from build123d import *

# Parameters (mm, degrees)
SKETCH_1_W          = 30
SKETCH_1_H          = 30
SKETCH_1_R          = 1.55
EXTRUDE_1_DEPTH     = 10
SKETCH_2_R          = 3.5
CUT_EXTRUDE_1_DEPTH = 3
SKETCH_3_W          = 6
SKETCH_3_H          = 15
EXTRUDE_3_DEPTH     = 3
SKETCH_5_W          = 1.5
SKETCH_5_H          = 0.7
CUT_EXTRUDE_3_DEPTH = 36
SKETCH_6_R          = 3
EXTRUDE_4_DEPTH     = 6


with BuildPart() as part:
    # 草图1 → 凸台-拉伸1 (new body)
    with BuildSketch(Plane(origin=(0, 0, 0), x_dir=(1, 0, 0), z_dir=(0, 1, 0))):
        Rectangle(SKETCH_1_W, SKETCH_1_H)
        with Locations(Location((-5, 5, 0), (0, 0, 270))):
            Circle(SKETCH_1_R, mode=Mode.SUBTRACT)
        with Locations(Location((5, 5, 0), (0, 0, 270))):
            Circle(SKETCH_1_R, mode=Mode.SUBTRACT)
        with Locations(Location((5, -5, 0), (0, 0, 270))):
            Circle(SKETCH_1_R, mode=Mode.SUBTRACT)
        with Locations(Location((-5, -5, 0), (0, 0, 270))):
            Circle(SKETCH_1_R, mode=Mode.SUBTRACT)
    extrude(amount=EXTRUDE_1_DEPTH)

    # 草图2 → 切除-拉伸1 (cut)
    with BuildSketch(Plane.XZ):
        with Locations(Location((-5, 5, 0), (0, 0, 270))):
            Circle(SKETCH_2_R)
        with Locations(Location((5, 5, 0), (0, 0, 270))):
            Circle(SKETCH_2_R)
        with Locations(Location((5, -5, 0), (0, 0, 270))):
            Circle(SKETCH_2_R)
        with Locations(Location((-5, -5, 0), (0, 0, 270))):
            Circle(SKETCH_2_R)
    extrude(amount=-CUT_EXTRUDE_1_DEPTH, mode=Mode.SUBTRACT)

    # 草图3 → 凸台-拉伸3 (add)
    with BuildSketch(Plane.XZ):
        with Locations((-12, 0)):
            Rectangle(SKETCH_3_W, SKETCH_3_H)
        with Locations((12, 0)):
            Rectangle(SKETCH_3_W, SKETCH_3_H)
    extrude(amount=EXTRUDE_3_DEPTH)

    # 草图5 → 切除-拉伸3 (cut, through all)
    with BuildSketch(Plane.ZY.offset(15)):
        with Locations((-6.75, -0.35)):
            Rectangle(SKETCH_5_W, SKETCH_5_H)
        with Locations((6.75, -0.35)):
            Rectangle(SKETCH_5_W, SKETCH_5_H)
    extrude(amount=-CUT_EXTRUDE_3_DEPTH, mode=Mode.SUBTRACT)

    # 草图6 → 凸台-拉伸4 (add)
    with BuildSketch(Plane.XZ):
        with Locations(Location((0, 0, 0), (0, 0, 270))):
            Circle(SKETCH_6_R)
    extrude(amount=EXTRUDE_4_DEPTH)


solid = part.part
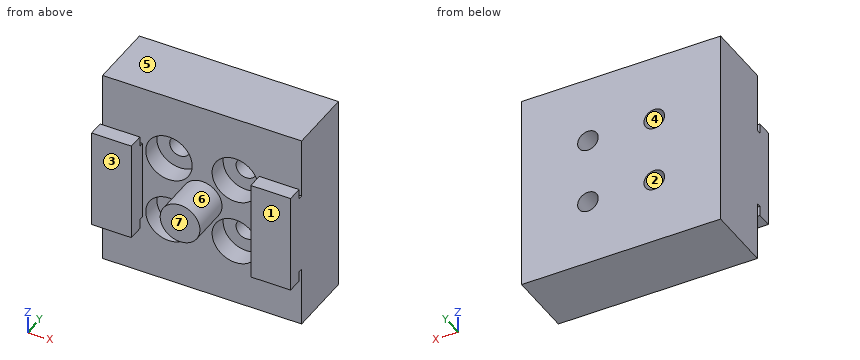
Design review of the part built by this model. Coordinates are the model's own, in mm. Face numbers are marked on the shaded views. A direction names the side the tool comes from. Round coordinates to 2 decimals unless told otherwise and drop trailing zeros. Write each loop counter-clockwise with the first axis right and the second up, starting at its lowest first coordinate (ties: lowest second). Pieces come first, ordered by that corner, then holes. Notation, with made-up numbers: M -39.5,-28 L -1.5,-28 A15 cw -1.5,-3 Z; hole C 1.5,67 d3. An arc over 180 degrees is marked long. One line per item, written item: value. Start each with the question number.
1. Draft analysis for pull direction Z (two halves, no side actions). For the marked faces 4, 5, 6 and 7, state which applies: pulls with the +Z half, pulls with the -Z half, needs draft (parallel to the pull), parting line crosses it, or undercut.
2. Take a section at A-A on z = -5. State the section outline as (x, y) points.
3. Clearance check with flat-ended pins moving along their axes: P1, Ø1.2, axis at x = -11.5, y = -2, coming from the -Z side; P2, Ø3, axis at x = -8, y = -3.5, coming from the +Z side; P3, Ø7.5, axis at x = -5, z = -6, coming from the -Y side; P4, Ø2.5, axis at x = 5, z = 5, coming from the -Y side. State where each tip first meets the part, or that it passes through.
4. To check wall thickness, follow probe 1 along Z at (x, y) = (5, 6.25); probe 2 along Z at (x, y) = (5, 1.45). State the ranges of each line that lie inside material, in increasing order. Write a range as from..to.
5. Take a section at C-C on y = 2. State the section outline as (x, z) points, then the cut area to 3 significant figures.
6. For the marked faces 1, 2 and 3, list the 3-axis set-ups (+Z, -Z, +X, -X, +Y, -Y) from which the entire face can be reached by the end or side of a thin tool; tool diameter is ignored.
7. Take a section at B-B on x = 5. State the section outline as (y, z) points.
8. Take a section at D-D on x = 0. State the section outline as (y, z) points.
Computed:
1. face 4: undercut
1. face 5: pulls with the +Z half
1. face 6: parting line crosses it
1. face 7: needs draft
2. outline: M -15,-3 L -9,-3 L -9,0 L -8.5,0 L -8.5,3 L -6.55,3 L -6.55,10 L -15,10 Z; M -3.45,3 L -1.5,3 L -1.5,0 L 1.5,0 L 1.5,3 L 3.45,3 L 3.45,10 L -3.45,10 Z; M 6.55,3 L 8.5,3 L 8.5,0 L 9,0 L 9,-3 L 15,-3 L 15,10 L 6.55,10 Z
3. P1: stops at z = -7.5
3. P2: stops at z = 7.5
3. P3: stops at y = 0
3. P4: passes through
4. probe 1: z = -15..-6.55, -3.45..3.45, 6.55..15
4. probe 2: z = -15..-8.5, -1.5..1.5, 8.5..15
5. outline: M -15,-15 L 15,-15 L 15,15 L -15,15 Z; hole C -5,-5 d7; hole C -5,5 d7; hole C 5,-5 d7; hole C 5,5 d7
5. area: 746 mm²
6. face 1: +Z, -Z, +X, -Y
6. face 2: +Y, -Y
6. face 3: +Z, -Z, -X, -Y
7. outline: M 0,-15 L 10,-15 L 10,-6.55 L 3,-6.55 L 3,-8.5 L 0,-8.5 Z; M 0,-1.5 L 3,-1.5 L 3,-3.45 L 10,-3.45 L 10,3.45 L 3,3.45 L 3,1.5 L 0,1.5 Z; M 0,8.5 L 3,8.5 L 3,6.55 L 10,6.55 L 10,15 L 0,15 Z
8. outline: M -6,-3 L 0,-3 L 0,-15 L 10,-15 L 10,15 L 0,15 L 0,3 L -6,3 Z
